Geometry check sheet. Reference: the model listing, model coordinates, mm. Give positions to 0.01 mm unless a question says otherwise; leave off trailing zeros. Use a Markdown table: item, result.
```python
from build123d import *

# Parameters (mm, degrees)
SKETCH1_W           = 158.75
SKETCH1_H           = 31.75
BOSS_EXTRUDE1_DEPTH = 4.064
SKETCH2_R           = 1.4478
CUT_EXTRUDE1_DEPTH  = 5.064
CHAMFER1_SIZE       = 1.143
SKETCH4_R           = 0.24003
CUT_EXTRUDE2_DEPTH  = 5.064
LPATTERN1_COUNT     = 10
LPATTERN1_PITCH     = 10.8204


with BuildPart() as part:
    # Sketch1 → Boss-Extrude1 (new body)
    with BuildSketch(Plane.XY):
        with Locations((47.727419355, 4.199193548)):
            Rectangle(SKETCH1_W, SKETCH1_H)
    extrude(amount=-BOSS_EXTRUDE1_DEPTH)

    # Sketch2 → Cut-Extrude1 (cut, through all)
    with BuildSketch(Plane.XY):
        with Locations((-18.947580645, 4.199193548)):
            Circle(SKETCH2_R)
        with Locations((114.402419355, 8.961693548)):
            Circle(SKETCH2_R)
    extrude(amount=-CUT_EXTRUDE1_DEPTH, mode=Mode.SUBTRACT)

    # Chamfer1
    chamfer1_edges = [part.edges().sort_by_distance(p)[0] for p in [
        (-20.395380645, 4.199193548, 0),
        (112.954619355, 8.961693548, 0),
    ]]
    chamfer(chamfer1_edges, length=CHAMFER1_SIZE)

    # Sketch4 → Cut-Extrude2 (cut, through all)
    with BuildSketch(Plane.XY):
        with Locations((-0.938980645, 4.199193548)):
            Circle(SKETCH4_R)
    cut_extrude2 = extrude(amount=-CUT_EXTRUDE2_DEPTH, mode=Mode.SUBTRACT)

    # LPattern1: Cut-Extrude2 ×10
    with Locations(*[(i * LPATTERN1_PITCH, 0, 0) for i in range(1, LPATTERN1_COUNT)]):
        add(cut_extrude2, mode=Mode.SUBTRACT)


solid = part.part
```
1) Mould release check, pull along Y, two halves, no side actions. Record for faces 1 (the flat face through (47, -11.676, -2)), 2 (the cylindrical face through (112.956, 9.025, -2.583)), 3 (the flat face through (47, 4, -4.064)), 4 (the cylindrical face through (-17.61, 3.64, -2.58)): pulls with the +Y half, pulls with the -Y half, needs draft (parallel to the pull), parting line crosses it, or undercut.
Working result:
| item | result |
|---|---|
| face 1 | pulls with the -Y half |
| face 2 | undercut |
| face 3 | needs draft |
| face 4 | undercut |
2) Material ranges on L1, parallel to X at y = 7, z = -0.15; L2, parallel to X at y = 9, z = -3.4, recorded low to high. Write a range as from..to.
Working result:
| item | result |
|---|---|
| L1 | x = -31.65..112.95, 115.85..127.1 |
| L2 | x = -31.65..112.96, 115.85..127.1 |
3) Depth check by flat-ended pin: P1, Ø5, axis at x = -2, y = 13, coming from the +Z side; P2, Ø2.5, axis at x = -18.95, y = 4.2, coming from the -Z side; P3, Ø3.5, axis at x = 114.4, y = 8.96, coming from the +Z side. Enter the tip coordinate at first touch or a pass-through.
Working result:
| item | result |
|---|---|
| P1 | stops at z = 0 |
| P2 | passes through |
| P3 | stops at z = -0.84 |
